Here's how the part is built. I have some questions about the finished solid (model axes, mm). A direction names the side the tool comes from. Give positions to 0.01 mm unless a question says otherwise; leave off trailing zeros. Loops run counter-clockwise (first coordinate to the right, second up) from the corner with the lowest first, then second, coordinate; pieces in that order, holes last. Notation, with made-up numbers: (60.5, 1) - (69.5, 1) arc R29 cw to (69.5, 23) - close; hole circle Ø11 at (-24.5, 26.5). An arc over 180 degrees is marked (long way). Return JSON: item names as keys, results as strings. Group by question number.
(1) If we section it at B-B (y = -18.25): Please give me the cut outline in (x, z), then the cut area to 3 significant figures.
(2) If we section it at A-A (z = -7): Please give me the cut outline in (x, y), then the cut area to 3 significant figures.
(3) I need wall thicknesses on probe 1 along Z at (x, y) = (-29.5, -5.75); probe 2 along Z at (x, y) = (-30, -8.75); probe 3 along X at (y, z) = (-11.75, 12). Which ranges of each line are inside material? Lowest first, please. Write a range as [from, to].
(4) If we section it at D-D (x = -44): Please give me the cut outline in (y, z).
(5) On a 3-axis mill with a long thin cutter (end or side, diameter ignored), from which of +Z, -Z, +X, -X, +Y, -Y can I reach the whole of each face in a straight line? I mean faces 5 (the flat face through (-15, -10, -11)), 6 (the cylindrical face through (-24.98, -9.86, 12.39)). Say none if no direction works.
(6) If we mould it in two halves opening along X, with no side actions, what happens to faces 1 (the cylindrical face through (-29.34, -9.86, 52.046)), 2 (the flat face through (-60, -10, 3)), 3 (the flat face through (-30, -10, -5.947)), 4 (the flat face through (-8, -10, -15.947))? For each: released by +X, released by -X, zero draft, split by the parting line, or undercut.
(7) If we section it at C-C (x = -30): Please give me the cut outline in (y, z).
(8) For P1, Ø5, axis at y = -15, z = -12.5, coming from the +X side; P2, Ø6, axis at x = -46, y = -6.5, coming from the +Z side; P3, Ø8, axis at y = -9.5, z = 34.5, coming from the +X side; P4, Ø19.5, axis at x = -30, z = 22.05, coming from the +Y side, each with a flat end and sliding along its axis, tell me the tip position at first contact or that it passes through.
```python
from build123d import *

# Parameters (mm, degrees)
F0_R     = 10.887967
F1_DEPTH = 20
F2_W     = 30
F2_H     = 10
F3_DEPTH = 20.001


with BuildPart() as f1:
    # F0 (on Front) → F1 (new body)
    with BuildSketch(Plane.XZ):
        with BuildLine():
            ThreePointArc((0, 22.053424), (-30, 52.053424), (-60, 22.053424))
            Line((-60, 22.053424), (-60, -15.946576))
            Line((-60, -15.946576), (0, -15.946576))
            Line((0, -15.946576), (0, 22.053424))
        make_face()
        with Locations((-30, 22.053424)):
            Circle(F0_R, mode=Mode.SUBTRACT)
    extrude(amount=F1_DEPTH)

    # F2 (on face) → F3 (cut, through all)
    with BuildSketch(Plane.XZ.offset(20)):
        with Locations((-30, -10.946576)):
            Rectangle(F2_W, F2_H)
    extrude(amount=-F3_DEPTH, mode=Mode.SUBTRACT)


solid = f1.part
```
Values:
{
 "1": {"outline": "(-60, -15.95) - (-45, -15.95) - (-45, -5.95) - (-15, -5.95) - (-15, -15.95) - (0, -15.95) - (0, 22.05) arc R30 ccw to (-60, 22.05) - close; hole circle Ø21.78 at (-30, 22.05)", "area": "3,020 mm2"},
 "2": {"outline": "(-60, -20) - (-45, -20) - (-45, 0) - (-60, 0) - close; (-15, -20) - (0, -20) - (0, 0) - (-15, 0) - close", "area": "600 mm2"},
 "3": {"probe 1": "[-5.95, 11.18], [32.93, 52.05]", "probe 2": "[-5.95, 11.17], [32.94, 52.05]", "probe 3": "[-60, -34.18], [-25.82, 0]"},
 "4": {"outline": "(-20, -5.95) - (0, -5.95) - (0, 48.59) - (-20, 48.59) - close"},
 "5": {"face 5": "-Z, +Y, -Y", "face 6": "+Y, -Y"},
 "6": {"face 1": "split by the parting line", "face 2": "released by -X", "face 3": "undercut", "face 4": "zero draft"},
 "7": {"outline": "(-20, -5.95) - (0, -5.95) - (0, 11.17) - (-20, 11.17) - close; (-20, 32.94) - (0, 32.94) - (0, 52.05) - (-20, 52.05) - close"},
 "8": {"P1": "x = 0", "P2": "z = 49.09", "P3": "x = -1.21", "P4": "through"}
}
